Answer from the drawing. Dimensions are ordinates in mm from the lowest x, y and z of the part. A direction names the side the tool comes from. Coordinates: 2 decimals unless noted, no trailing zeros. Order: outer loops, then holes, each group sorted by start corner. A loop starts at its lowest first (then second) coordinate and runs counter-clockwise, first axis right, second up. Notation, with made-up numbers: (-38.75, -23) -> (-16.75, -23) arc R7 ccw to (-16.75, -11) -> close; hole circle Ø1 at (4.5, 75.25). An arc over 180 degrees is marked (long way). Answer in a Markdown table with one row per item.
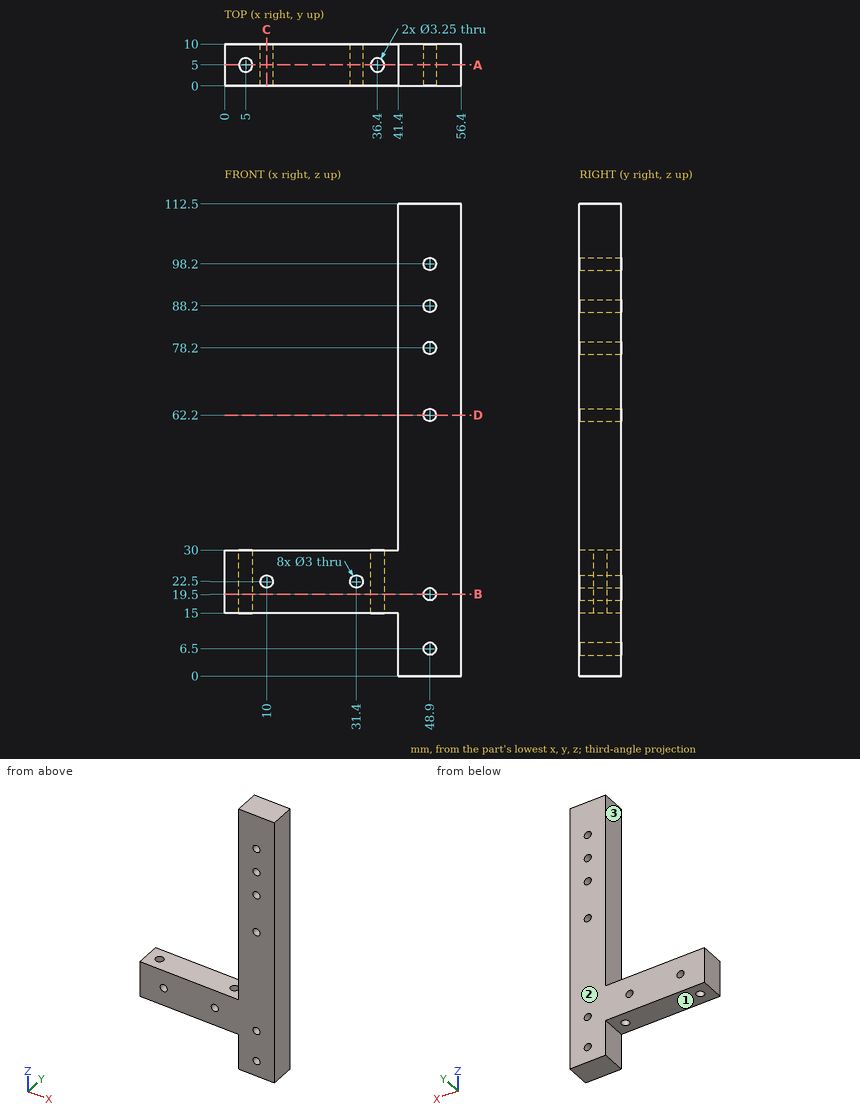
(1) A cutting plane is placed at A-A, the plane y = 5. Count the separate pieces of the cut face and the enclosed holes in it, then the cut area to 3 significant figures.
Check values:
| item | result |
|---|---|
| separate pieces | 3 |
| enclosed holes | 8 |
| area | 2,150 mm² |
(2) A cutting plane is placed at B-B, the plane z = 19.5. Determine the outline of the cut face in (x, y) (3 decimals).
Check values:
| item | result |
|---|---|
| outline | (0, 0) -> (47.4, 0) -> (47.4, 10) -> (0, 10) -> close; (50.4, 0) -> (56.4, 0) -> (56.4, 10) -> (50.4, 10) -> close; hole circle Ø3.25 at (5, 5); hole circle Ø3.25 at (36.4, 5) |
(3) Which of the six approach directions +Z, -Z, +X, -X, +Y, -Y give full straight-line access (tool end or side, diameter ignored) to the marked faces 1, 2 and 3?
Check values:
| item | result |
|---|---|
| face 1 | -Z, -X, +Y, -Y |
| face 2 | +Z, -Z, +X, -X, +Y |
| face 3 | +Z, -X, +Y, -Y |
(4) A cutting plane is placed at D-D, the plane z = 62.2. Determine the outline of the cut face in (x, y).
Check values:
| item | result |
|---|---|
| outline | (41.4, 0) -> (47.4, 0) -> (47.4, 10) -> (41.4, 10) -> close; (50.4, 0) -> (56.4, 0) -> (56.4, 10) -> (50.4, 10) -> close |
(5) A cutting plane is placed at C-C, the plane x = 10. Determine the outline of the cut face in (y, z).
Check values:
| item | result |
|---|---|
| outline | (0, 15) -> (10, 15) -> (10, 21) -> (0, 21) -> close; (0, 24) -> (10, 24) -> (10, 30) -> (0, 30) -> close |
(6) Find the intervals of material crossed by line 1 along X through (y, z) = (7, 19.5); line 2 along X through (y, z) = (5, 78.2); line 3 along X through (y, z) = (8.75, 49.5), in increasing order. Write a range as from..to.
Check values:
| item | result |
|---|---|
| line 1 | 0..47.4, 50.4..56.4 |
| line 2 | 41.4..47.4, 50.4..56.4 |
| line 3 | 41.4..56.4 |
(7) Flat-ended cylindrical pins translate along their axes: pin 1 (1.8 mm diameter, centred on x = 10, z = 22.5, fed in from +Y); pin 2 (5 mm diameter, centred on y = 5, z = 58, fed in from -X); pin 3 (5 mm diameter, centred on x = 12.5, y = 7, fed in from +Z); pin 4 (5 mm diameter, centred on x = 48.9, z = 88.2, fed in from -Y). Find the tip coordinate at first contact, or state that the pin passes through.
Check values:
| item | result |
|---|---|
| pin 1 | through |
| pin 2 | x = 41.4 |
| pin 3 | z = 30 |
| pin 4 | y = 0 |
